Verification items for this drawing (mm, ordinates from the low corner). Round coordinates to 2 decimals unless told otherwise and drop trailing zeros. Order: outer loops, then holes, each group sorted by start corner. A loop starts at its lowest first (then second) coordinate and runs counter-clockwise, first axis right, second up. Notation, with made-up numbers: M -21.5,1 L -6.5,1 A18 ccw -6.5,20 Z; hole C 68.5,-21 d7. An arc over 180 degrees is marked long. One line per item, written item: value. Start each with the question number.
(1) Cross-section at C-C, the plane z = 32. Enter the section's corners in (x, y), and give its area (3 significant figures).
(2) Cross-section at A-A, the plane y = 5.5. Enter the section's corners in (x, z).
(3) Depth check by flat-ended pin: pin 1 Ø3.5 at (x, y) = (15, 5.5) entering from +Z. Enter the tip coordinate at first touch or a pass-through.
(4) Cross-section at B-B, the plane x = 24. Enter the section's corners in (y, z), and give its area (3 significant figures).
(5) Release check for a two-part mould opening along X. For the marked faces 1, 2 and 3 record: released by +X, released by -X, zero draft, split by the parting line, or undercut.
(6) Thickness scan on L1, parallel to Z at x = 24, y = 2.75; L2, parallel to X at y = 2, z = 9; L3, parallel to X at y = 4.5, z = 32. Record the ranges inside material, lowest first.
(7) Cross-section at D-D, the plane z = 20.5. Enter the section's corners in (x, y), and give its area (3 significant figures).
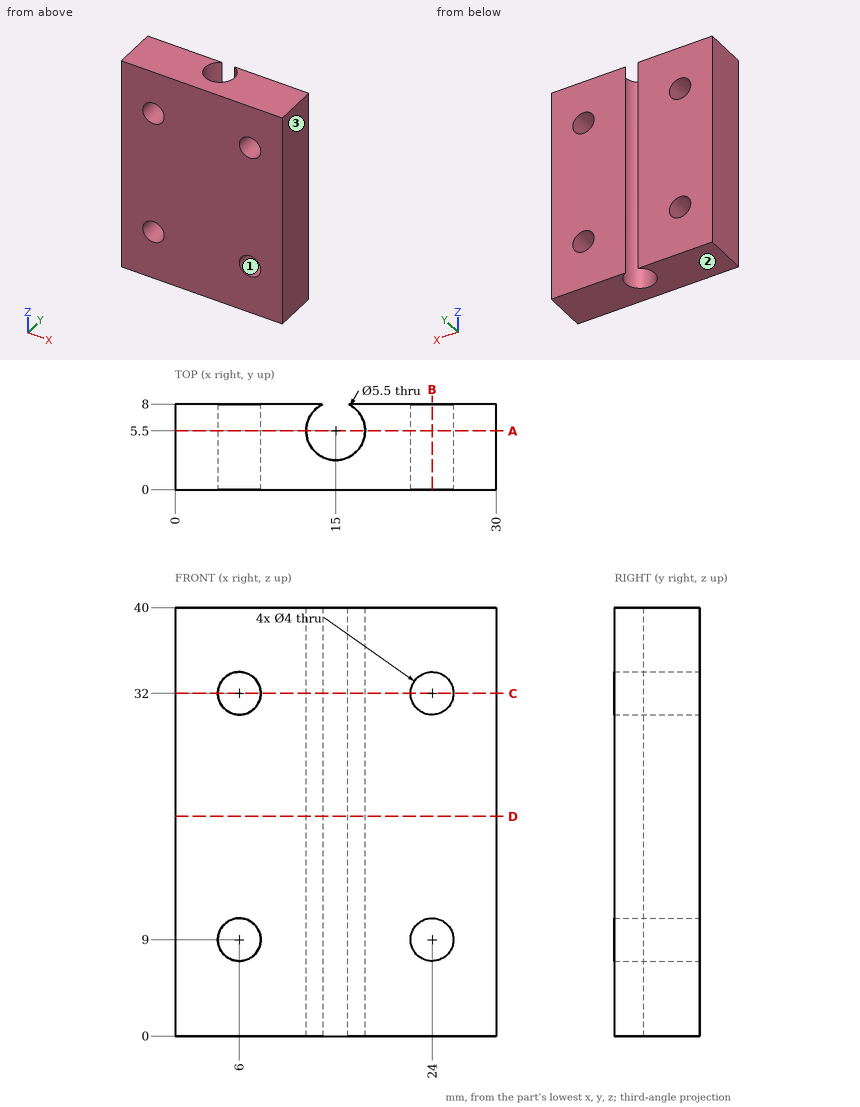
Values found:
1. outline: M 0,0 L 4,0 L 4,8 L 0,8 Z; M 8,0 L 22,0 L 22,8 L 16.15,8 A2.75 cw long 13.85,8 L 8,8 Z; M 26,0 L 30,0 L 30,8 L 26,8 Z
1. area: 153 mm^2
2. outline: M 0,0 L 12.25,0 L 12.25,40 L 0,40 Z; M 17.75,0 L 30,0 L 30,40 L 17.75,40 Z; hole C 6,9 d4; hole C 6,32 d4; hole C 24,9 d4; hole C 24,32 d4
3. pin 1: through
4. outline: M 0,0 L 8,0 L 8,7 L 0,7 Z; M 0,11 L 8,11 L 8,30 L 0,30 Z; M 0,34 L 8,34 L 8,40 L 0,40 Z
4. area: 256 mm^2
5. face 1: undercut
5. face 2: zero draft
5. face 3: released by +X
6. L1: 0 to 7, 11 to 30, 34 to 40
6. L2: 0 to 4, 8 to 22, 26 to 30
6. L3: 0 to 4, 8 to 12.44, 17.56 to 22, 26 to 30
7. outline: M 0,0 L 30,0 L 30,8 L 16.15,8 A2.75 cw long 13.85,8 L 0,8 Z
7. area: 217 mm^2
